from build123d import *

# Parameters (mm, degrees)
F0_W     = 105
F0_H     = 30
F0_R     = 1.5
F0_W_2   = 9
F0_H_2   = 11
F0_W_3   = 32
F0_H_3   = 13
F0_W_4   = 19
F0_H_4   = 15
F1_DEPTH = 1.25
F2_R     = 5
F3_SIZE  = 1


with BuildPart() as f1:
    # F0 (on Front) → F1 (new body)
    with BuildSketch(Plane.XZ):
        with Locations((0.5, -4.707695)):
            Rectangle(F0_W, F0_H)
        with Locations((-48, -16.207695)):
            Circle(F0_R, mode=Mode.SUBTRACT)
        with Locations((-40.5, -7.207695)):
            Rectangle(F0_W_2, F0_H_2, mode=Mode.SUBTRACT)
        with Locations((-16, -6.207695)):
            Rectangle(F0_W_3, F0_H_3, mode=Mode.SUBTRACT)
        with Locations((49, -16.207695)):
            Circle(F0_R, mode=Mode.SUBTRACT)
        with Locations((33.5, -5.207695)):
            Rectangle(F0_W_4, F0_H_4, mode=Mode.SUBTRACT)
        with Locations((-48, 6.792305)):
            Circle(F0_R, mode=Mode.SUBTRACT)
        with Locations((49, 6.792305)):
            Circle(F0_R, mode=Mode.SUBTRACT)
    extrude(amount=F1_DEPTH)

    # F2
    f2_edges = [f1.edges().sort_by_distance(p)[0] for p in [
        (53, -0.625, 10.292305),
        (53, -0.625, -19.707695),
        (-52, -0.625, -19.707695),
        (-52, -0.625, 10.292305),
    ]]
    fillet(f2_edges, radius=F2_R)

    # F3
    f3_edges = [f1.edges().sort_by_distance(p)[0] for p in [
        (47.5, -1.25, 6.792305),
        (47.5, -1.25, -16.207695),
        (-49.5, -1.25, -16.207695),
        (-49.5, -1.25, 6.792305),
    ]]
    chamfer(f3_edges, length=F3_SIZE)


solid = f1.part
The model under review builds one solid part; all positions refer to its coordinate system, in mm. Give positions to 0.01 mm unless a question says otherwise; leave off trailing zeros. Write each loop counter-clockwise with the first axis right and the second up, starting at its lowest first coordinate (ties: lowest second). Pieces come first, ordered by that corner, then holes.
1. Draft analysis for pull direction X (two halves, no side actions). For faces 1 (the cylindrical face through (51.496, -0.634, 8.866)), 2 (the cylindrical face through (-50.574, -0.634, 8.789)), 3 (the flat face through (0, -1.25, 2)), state which applies: +X half, -X half, draft (parallel to the pull), parting line (faces both ways), or undercut.
2. Add section B-B, the plane y = -0.8. Write out the cut boundary in (x, z).
3. Add section D-D, the plane x = 35. Write out the cut boundary in (y, z), plus the area to 4 significant figures.
4. Add section C-C, the plane x = 49. Write out the cut boundary in (y, z).
5. Add section A-A, the plane x = -9. Write out the cut boundary in (y, z), plus the area to 4 significant figures.
6. Wall thickness on L1, parallel to X at y = -0.35, z = -10.5; L2, parallel to Z at x = -20, y = -0.8; L3, parallel to Z at x = -48, y = -0.15: over which ranges is each line inside the solid? List them lowest first.
Worked answers:
1. face 1: +X half
1. face 2: -X half
1. face 3: draft
2. outline: (-52, -14.71) arc R5 ccw to (-47, -19.71) - (48, -19.71) arc R5 ccw to (53, -14.71) - (53, 5.29) arc R5 ccw to (48, 10.29) - (-47, 10.29) arc R5 ccw to (-52, 5.29) - close; hole circle Ø4.1 at (-48, -16.21); hole circle Ø4.1 at (-48, 6.79); hole (-45, -12.71) - (-36, -12.71) - (-36, -1.71) - (-45, -1.71) - close; hole (-32, -12.71) - (0, -12.71) - (0, 0.29) - (-32, 0.29) - close; hole (24, -12.71) - (43, -12.71) - (43, 2.29) - (24, 2.29) - close; hole circle Ø4.1 at (49, -16.21); hole circle Ø4.1 at (49, 6.79)
3. outline: (-1.25, -19.71) - (0, -19.71) - (0, -12.71) - (-1.25, -12.71) - close; (-1.25, 2.29) - (0, 2.29) - (0, 10.29) - (-1.25, 10.29) - close
3. area: 18.75 mm2
4. outline: (-1.25, -19.61) - (0, -19.61) - (0, -17.71) - (-0.25, -17.71) - (-1.25, -18.71) - close; (-1.25, -13.71) - (-0.25, -14.71) - (0, -14.71) - (0, 5.29) - (-0.25, 5.29) - (-1.25, 4.29) - close; (-1.25, 9.29) - (-0.25, 8.29) - (0, 8.29) - (0, 10.19) - (-1.25, 10.19) - close
5. outline: (-1.25, -19.71) - (0, -19.71) - (0, -12.71) - (-1.25, -12.71) - close; (-1.25, 0.29) - (0, 0.29) - (0, 10.29) - (-1.25, 10.29) - close
5. area: 21.25 mm2
6. L1: x = -52 to -45, -36 to -32, 0 to 24, 43 to 53
6. L2: z = -19.71 to -12.71, 0.29 to 10.29
6. L3: z = -19.61 to -17.71, -14.71 to 5.29, 8.29 to 10.19
